```python
from build123d import *

# Parameters (mm, degrees)
SKETCH1_R           = 10
BOSS_EXTRUDE1_DEPTH = 2.5
SKETCH2_R           = 15
SKETCH2_R_2         = 10
BOSS_EXTRUDE2_DEPTH = 15
SKETCH3_R           = 5
CUT_EXTRUDE1_DEPTH  = 82.403700776
BOSS_EXTRUDE3_START = 9.5
SKETCH4_R           = 10
SKETCH4_R_2         = 6
BOSS_EXTRUDE3_DEPTH = 3


with BuildPart() as part:
    # Sketch1 → Boss-Extrude1 (new, symmetric)
    with BuildSketch(Plane(origin=(0, 0, 0), x_dir=(1, 0, 0), z_dir=(0, 1, 0))):
        with BuildLine():
            Line((12.5, 12.5), (12.5, 26.25))
            ThreePointArc((12.5, 26.25), (0, 38.75), (-12.5, 26.25))
            Line((-12.5, 26.25), (-12.5, 12.5))
            Line((-12.5, 12.5), (-62.5, 7.5))
            ThreePointArc((-62.5, 7.5), (-70, 0), (-62.5, -7.5))
            Line((-62.5, -7.5), (-12.5, -12.5))
            Line((-12.5, -12.5), (-12.5, -26.25))
            ThreePointArc((-12.5, -26.25), (0, -38.75), (12.5, -26.25))
            Line((12.5, -26.25), (12.5, -12.5))
            Line((12.5, -12.5), (62.5, -7.5))
            ThreePointArc((62.5, -7.5), (70, 0), (62.5, 7.5))
            Line((62.5, 7.5), (12.5, 12.5))
        make_face()
        with Locations(Location((0, 0, 0), (0, 0, 270))):
            Circle(SKETCH1_R, mode=Mode.SUBTRACT)
    extrude(amount=BOSS_EXTRUDE1_DEPTH, both=True)

    # Sketch2 → Boss-Extrude2 (add)
    with BuildSketch(Plane(origin=(0, 2.5, 0), x_dir=(1, 0, 0), z_dir=(0, 1, 0))):
        with Locations(Location((0, 0, 0), (0, 0, 90))):
            Circle(SKETCH2_R)
        with Locations(Location((0, 0, 0), (0, 0, 270))):
            Circle(SKETCH2_R_2, mode=Mode.SUBTRACT)
    extrude(amount=BOSS_EXTRUDE2_DEPTH)

    # Sketch3 → Cut-Extrude1 (cut, through all)
    with BuildSketch(Plane(origin=(0, 2.5, 0), x_dir=(1, 0, 0), z_dir=(0, 1, 0))):
        with Locations(Location((42.5, 0, 0), (0, 0, 270))):
            Circle(SKETCH3_R)
        with Locations(Location((-42.5, 0, 0), (0, 0, 270))):
            Circle(SKETCH3_R)
    extrude(amount=-CUT_EXTRUDE1_DEPTH, mode=Mode.SUBTRACT)

    # Sketch4 → Boss-Extrude3 (add)
    with BuildSketch(Plane(origin=(0, 0, 0), x_dir=(1, 0, 0), z_dir=(0, 1, 0)).offset(BOSS_EXTRUDE3_START)):
        with Locations(Location((0, 0, 0), (0, 0, 270))):
            Circle(SKETCH4_R)
        with Locations(Location((0, 0, 0), (0, 0, 270))):
            Circle(SKETCH4_R_2, mode=Mode.SUBTRACT)
    extrude(amount=BOSS_EXTRUDE3_DEPTH)


solid = part.part
```
The listing builds one solid part. Answer for the finished solid, in the listing's coordinates (mm). A direction names the side the tool comes from. Coordinates: 2 decimals unless noted, no trailing zeros. Order: outer loops, then holes, each group sorted by start corner. A loop starts at its lowest first (then second) coordinate and runs counter-clockwise, first axis right, second up. Notation, with made-up numbers: M 33,36.25 L 38,36.25 A30 ccw 38,65.25 Z; hole C -8,-8.75 d1. An arc over 180 degrees is marked long. Answer as a JSON object with one key per item and string values. Group by question number.
1. Section B-B on y = -0.5 is taken. Write down the section's boundary in (x, z), then the cut area to 3 significant figures.
2. Section D-D on x = 42.5 is taken. Write down the section's boundary in (y, z).
3. Determine the mould class of faces 1 (the flat face through (12.5, 0, -19)), 2 (the flat face through (-12.5, 0, -19)), 3 (the cylindrical face through (-9.76, 3.42, -2.17)) for opening direction X: released by +X, released by -X, zero draft, split by the parting line, or undercut.
4. A tool of negligible diameter and unlimited length cuts with its end or side. For faces 4 (the flat face through (-12.5, 0, 19)), 5 (the cylindrical face through (-9.76, 14.96, -2.17)), 6 (the flat face through (12.5, 0, 19)), from which of +Z, -Z, +X, -X, +Y, -Y can it reach the whole face along a straight path? Write none if from no direction.
5. Section A-A on x = 0 is taken. Write down the section's boundary in (y, z), then the cut area to 4 significant figures.
6. Flat-ended cylindrical pins translate along their axes: P1, Ø16, axis at x = -42.5, z = 0, coming from the +Y side; P2, Ø2.5, axis at y = -1, z = -21, coming from the -X side; P3, Ø4, axis at y = 1, z = -19, coming from the +X side. Find the tip coordinate at first contact, or state that the pin passes through.
7. Straight lines are drawn through the part: line 1 (X direction, y = 1, z = 0); line 2 (X direction, y = 14.2, z = 0); line 3 (Y direction, x = -4, z = 9). For each, find the intervals that lie inside material, in ascending order.
8. Section C-C on y = 6.5 is taken. Write down the section's boundary in (x, z), then the cut area to 3 significant figures.
Values follow:
{
 "1": {"outline": "M -62.5,-7.5 L -12.5,-12.5 L -12.5,-26.25 A12.5 ccw 12.5,-26.25 L 12.5,-12.5 L 62.5,-7.5 A7.5 ccw 62.5,7.5 L 12.5,12.5 L 12.5,26.25 A12.5 ccw -12.5,26.25 L -12.5,12.5 L -62.5,7.5 A7.5 ccw Z; hole C -42.5,0 d10; hole C 0,0 d20; hole C 42.5,0 d10", "area": "3,510 mm2"},
 "2": {"outline": "M -2.5,-9.5 L 2.5,-9.5 L 2.5,-5 L -2.5,-5 Z; M -2.5,5 L 2.5,5 L 2.5,9.5 L -2.5,9.5 Z"},
 "3": {"face 1": "released by +X", "face 2": "released by -X", "face 3": "undercut"},
 "4": {"face 4": "+Z, -X, +Y, -Y", "face 5": "+Y", "face 6": "+Z, +X, +Y, -Y"},
 "5": {"outline": "M -2.5,-38.75 L 2.5,-38.75 L 2.5,-15 L 17.5,-15 L 17.5,-10 L 12.5,-10 L 12.5,-6 L 9.5,-6 L 9.5,-10 L -2.5,-10 Z; M -2.5,10 L 9.5,10 L 9.5,6 L 12.5,6 L 12.5,10 L 17.5,10 L 17.5,15 L 2.5,15 L 2.5,38.75 L -2.5,38.75 Z", "area": "461.5 mm2"},
 "6": {"P1": "y = 2.5", "P2": "x = -12.5", "P3": "x = 12.5"},
 "7": {"line 1": "-70 to -47.5, -37.5 to -10, 10 to 37.5, 47.5 to 70", "line 2": "-15 to -10, 10 to 15", "line 3": "9.5 to 12.5"},
 "8": {"outline": "C 0,0 d30; hole C 0,0 d20", "area": "393 mm2"}
}
